Check sheet for the modelled part. Datum: model origin and axes. Units: mm. Give positions to 0.01 mm unless a question says otherwise; leave off trailing zeros. Order: outer loops, then holes, each group sorted by start corner. A loop starts at its lowest first (then second) coordinate and runs counter-clockwise, first axis right, second up.
```python
from build123d import *

# Parameters (mm, degrees)
BOSS_EXTRUDE1_DEPTH      = 18.5
BOSS_EXTRUDE1_DEPTH_BACK = 18.5
SKETCH1_R                = 0.3


with BuildPart() as part:
    # Sketch1 → Boss-Extrude1 (new, two sides: drawn at the far end of the back side and taken through both)
    with BuildSketch(Plane.XY.offset(-BOSS_EXTRUDE1_DEPTH_BACK)):
        Polygon((-1.955677856, 1.191654646), (2.044322144, 1.191654646), (2.963241063, -1.294831841), (-3.036758937, -1.294831841), align=None)
        with Locations((2.256164177, -0.813020011)):
            Circle(SKETCH1_R, mode=Mode.SUBTRACT)
        with Locations(Location((-2.329682051, -0.813020011, 0), (0, 0, 180))):
            Circle(SKETCH1_R, mode=Mode.SUBTRACT)
    extrude(amount=BOSS_EXTRUDE1_DEPTH + BOSS_EXTRUDE1_DEPTH_BACK)


solid = part.part
```
(1) Release check for a two-part mould opening along X. For faces 1 (the face through (-2.504, -0.069, -0.259)), 2 (the face through (0, 0, -18.5)), 3 (the face through (2.497, -0.034, -0.259)) record: released by +X, released by -X, zero draft, split by the parting line, or undercut.
Response values:
face 1: released by -X
face 2: zero draft
face 3: released by +X
(2) Material ranges on L1, parallel to Y at x = -2.25, z = -4.5; L2, parallel to X at y = 0.25, z = 8; L3, parallel to X at y = 0.9, z = -15, recorded low to high.
Response values:
L1: y = -1.29 to -1.1, -0.52 to 0.51
L2: x = -2.37 to 2.39
L3: x = -2.08 to 2.15
(3) Cross-section at B-B on y = 0.7. Enter the section's corners in (x, z), then the cut area to 3 significant figures.
Response values:
outline: (-2.17, -18.5) - (2.23, -18.5) - (2.23, 18.5) - (-2.17, 18.5) - close
area: 163 mm2
(4) Cross-section at A-A on z = -1.5. Enter the section's corners in (x, y).
Response values:
outline: (-3.04, -1.29) - (2.96, -1.29) - (2.04, 1.19) - (-1.96, 1.19) - close; hole circle Ø0.6 at (-2.33, -0.81); hole circle Ø0.6 at (2.26, -0.81)
